Work out the finished part from the listing and answer in its coordinate system (mm). Face numbers are marked on the shaded views. Give positions to 0.01 mm unless a question says otherwise; leave off trailing zeros. Order: outer loops, then holes, each group sorted by start corner. A loop starts at its lowest first (then second) coordinate and runs counter-clockwise, first axis right, second up. Notation, with made-up numbers: M -40,-2 L -5,-2 A14 ccw -5,18 Z; hole C 10,13 d2. An arc over 180 degrees is marked long. One line per item, written item: value.
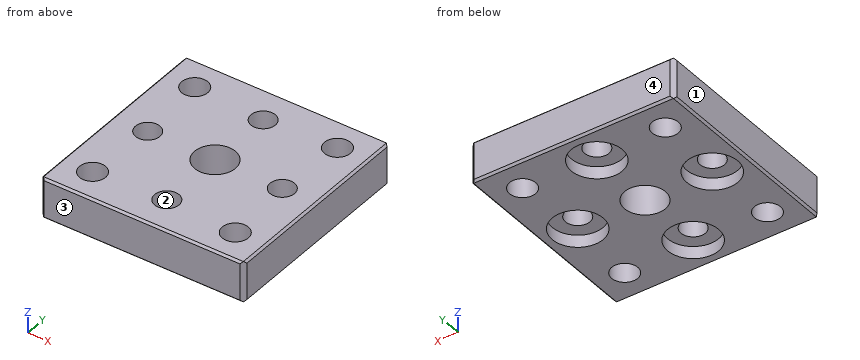
from build123d import *

# Parameters (mm, degrees)
SKETCH1_W                = 50
SKETCH1_H                = 50
BOSS_EXTRUDE1_DEPTH      = 5
M6_CLEARANCE_HOLE1_D     = 6.4
CUT_EXTRUDE1_REACH       = 38.742
SKETCH5_R                = 5
CHAMFER1_SIZE            = 1
CHAMFER2_SIZE            = 0.5
F_6_0_6_DIAMETER_HOLE1_D = 6
SKETCH12_R               = 6.25
CUT_EXTRUDE2_DEPTH       = 3


with BuildPart() as part:
    # Sketch1 → Boss-Extrude1 (new, symmetric)
    with BuildSketch(Plane.XY):
        Rectangle(SKETCH1_W, SKETCH1_H)
    extrude(amount=BOSS_EXTRUDE1_DEPTH, both=True)

    # M6 Clearance Hole1 (through all)
    with Locations(Plane.XY.offset(5)):
        with Locations((-17.5, 17.5), (17.5, 17.5), (17.5, -17.5), (-17.5, -17.5)):
            Hole(M6_CLEARANCE_HOLE1_D / 2)

    # Sketch5 → Cut-Extrude1 (cut, up to next)
    with BuildSketch(Plane.XY.offset(5), mode=Mode.PRIVATE) as cut_extrude1_sk1:
        Circle(SKETCH5_R)
    cut_extrude1_tool1 = extrude(cut_extrude1_sk1.sketch, amount=-CUT_EXTRUDE1_REACH, mode=Mode.PRIVATE) & part.part
    add(cut_extrude1_tool1.solids().sort_by_distance((0, 0, 5))[0], mode=Mode.SUBTRACT)

    # Chamfer1
    chamfer1_edges = [part.edges().sort_by_distance(p)[0] for p in [
        (25, -25, 0),
        (-25, -25, 0),
        (-25, 25, 0),
        (25, 25, 0),
    ]]
    chamfer(chamfer1_edges, length=CHAMFER1_SIZE)

    # Chamfer2
    chamfer2_edges = [part.edges().sort_by_distance(p)[0] for p in [
        (0, -25, 5),
        (0, -25, -5),
        (0, 25, -5),
        (0, 25, 5),
        (25, 0, -5),
        (25, 0, 5),
        (-25, 0, -5),
        (-25, 0, 5),
    ]]
    chamfer(chamfer2_edges, length=CHAMFER2_SIZE - 0.0001)  # a hair under: the kernel refuses the full size

    # Ø6.0 (6) Diameter Hole1 (through all)
    with Locations(Plane(origin=(0, 0, -5), x_dir=(-1, 0, 0), z_dir=(0, 0, -1))):
        with Locations((-16.5, 0), (0, 16.5), (16.5, 0), (0, -16.5)):
            Hole(F_6_0_6_DIAMETER_HOLE1_D / 2)

    # Sketch12 → Cut-Extrude2 (cut)
    with BuildSketch(Plane(origin=(0, 0, -5), x_dir=(-1, 0, 0), z_dir=(0, 0, -1))):
        with Locations((16.5, 0)):
            Circle(SKETCH12_R)
        with Locations((0, -16.5)):
            Circle(SKETCH12_R)
        with Locations((-16.5, 0)):
            Circle(SKETCH12_R)
        with Locations((0, 16.5)):
            Circle(SKETCH12_R)
    extrude(amount=-CUT_EXTRUDE2_DEPTH, mode=Mode.SUBTRACT)


solid = part.part
(1) Find the intervals of material crossed by probe 1 along Y at (x, z) = (-20, 1.5); probe 2 along X at (y, z) = (-16, -3.25); probe 3 along X at (y, z) = (1.5, -3.75), in increasing order. Write a range as from..to.
Findings:
probe 1: y = -25..-19.5, -15.5..15.5, 19.5..25
probe 2: x = -25..-20.33, -14.67..-6.23, 6.23..14.67, 20.33..25
probe 3: x = -25..-22.57, -10.43..-4.77, 4.77..10.43, 22.57..25
(2) Given P1, Ø11, axis at x = 0, y = -16.5, coming from the -Z side, flat-ended and moving along its own axis, determine where the tip first touches the part or whether it passes through.
Findings:
P1: stops at z = -2
(3) Determine the mould class of the marked faces 1, 2, 3 and 4 for opening direction Y: pulls with the +Y half, pulls with the -Y half, needs draft (parallel to the pull), parting line crosses it, or undercut.
Findings:
face 1: needs draft
face 2: undercut
face 3: pulls with the -Y half
face 4: pulls with the +Y half
(4) Section B-B, the plane x = 16 is taken. Give the vertices of the cut face in (y, z).
Findings:
outline: M -25,-4.5 L -24.5,-5 L -20.33,-5 L -20.33,5 L -24.5,5 L -25,4.5 Z; M -14.67,-5 L -6.23,-5 L -6.23,-2 L -2.96,-2 L -2.96,5 L -14.67,5 Z; M 2.96,-2 L 6.23,-2 L 6.23,-5 L 14.67,-5 L 14.67,5 L 2.96,5 Z; M 20.33,-5 L 24.5,-5 L 25,-4.5 L 25,4.5 L 24.5,5 L 20.33,5 Z
(5) Section A-A, the plane z = -3.25 is taken. Give the number of separate pieces and of enclosed holes in the cut face, then the cut area to 3 significant figures.
Findings:
separate pieces: 1
enclosed holes: 9
area: 1,800 mm^2
(6) Section D-D, the plane y = -11.5 is taken. Give the vertices of the cut face in (x, z).
Findings:
outline: M -25,-4.5 L -24.5,-5 L -3.75,-5 L -3.75,-2 L 3.75,-2 L 3.75,-5 L 24.5,-5 L 25,-4.5 L 25,4.5 L 24.5,5 L -24.5,5 L -25,4.5 Z
(7) Section C-C, the plane y = 2 is taken. Give the vertices of the cut face in (x, z).
Findings:
outline: M -25,-4.5 L -24.5,-5 L -22.42,-5 L -22.42,-2 L -18.74,-2 L -18.74,5 L -24.5,5 L -25,4.5 Z; M -14.26,-2 L -10.58,-2 L -10.58,-5 L -4.58,-5 L -4.58,5 L -14.26,5 Z; M 4.58,-5 L 10.58,-5 L 10.58,-2 L 14.26,-2 L 14.26,5 L 4.58,5 Z; M 18.74,-2 L 22.42,-2 L 22.42,-5 L 24.5,-5 L 25,-4.5 L 25,4.5 L 24.5,5 L 18.74,5 Z
